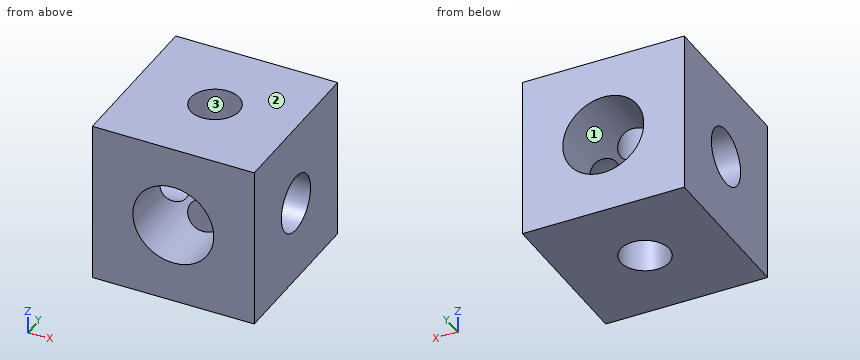
from build123d import *

# Parameters (mm, degrees)
F0_W     = 20
F0_H     = 20
F1_DEPTH = 20
F2_R     = 3
F3_DEPTH = 25
F4_R     = 3.5
F5_DEPTH = 25
F6_R     = 5
F7_DEPTH = 25


with BuildPart() as f1:
    # F0 (on Front) → F1 (new body)
    with BuildSketch(Plane.XZ):
        with Locations((15.513396, -6.90791)):
            Rectangle(F0_W, F0_H)
    extrude(amount=F1_DEPTH)

    # F2 (on face) → F3 (cut)
    with BuildSketch(Plane.XY.offset(3.09209)):
        with Locations((15.513396, -10)):
            Circle(F2_R)
    extrude(amount=-F3_DEPTH, mode=Mode.SUBTRACT)

    # F4 (on face) → F5 (cut)
    with BuildSketch(Plane.YZ.offset(25.513396)):
        with Locations((-10, -6.90791)):
            Circle(F4_R)
    extrude(amount=-F5_DEPTH, mode=Mode.SUBTRACT)

    # F6 (on face) → F7 (cut)
    with BuildSketch(Plane.XZ.offset(20)):
        with Locations((15.513396, -6.90791)):
            Circle(F6_R)
    extrude(amount=-F7_DEPTH, mode=Mode.SUBTRACT)


solid = f1.part
The model under review builds one solid part; all positions refer to its coordinate system, in mm. Face numbers are marked on the shaded views. Give positions to 0.01 mm unless a question says otherwise; leave off trailing zeros. Order: outer loops, then holes, each group sorted by start corner. A loop starts at its lowest first (then second) coordinate and runs counter-clockwise, first axis right, second up. Notation, with made-up numbers: M 80.5,70 L 111.5,70 A18 ccw 111.5,94 Z; hole C 44.5,-32.5 d11. An arc over 180 degrees is marked long. Use one line per item in the form item = value. Start each with the question number.
Item 1: To check wall thickness, follow line 1 along X through (y, z) = (-10, 1.75); line 2 along X through (y, z) = (-4.75, -6.75); line 3 along Z through (x, y) = (12.75, -13.75). State the ranges of each line that lie inside material, in increasing order. Write a range as from..to.
Item 2: Insertion check: pin 1 Ø7 at (x, y) = (15.51, -10) entering from -Z; pin 2 Ø8 at (x, z) = (15.51, -6.91) entering from -Y. Each pin has a flat end and moves straight along its axis. Give the tip position at first contact, or say it passes through.
Item 3: We need section A-A on y = -10. Give the boundary of the cut face in (x, z).
Item 4: We need section D-D on y = -7.5. Give the boundary of the cut face in (x, z).
Item 5: The part is to be moulded in two halves that separate along Z. For the marked faces 1, 2 and 3, say which applies: pulls with the +Z half, pulls with the -Z half, needs draft (parallel to the pull), parting line crosses it, or undercut.
Item 6: We need section C-C on z = -2.5. Give the boundary of the cut face in (x, y).
Item 7: We need section B-B on x = 17.75. Give the boundary of the cut face in (y, z), plus the area to 3 significant figures.
Completed:
q1.line_1 = 5.51..12.51, 18.51..25.51
q1.line_2 = 5.51..10.52, 20.51..25.51
q1.line_3 = -16.91..-11.07, -2.74..3.09
q2.pin_1 = -16.91
q2.pin_2 = through
q3.outline = M 5.51,-16.91 L 12.51,-16.91 L 12.51,-10.91 A5 cw 11.94,-10.41 L 5.51,-10.41 Z; M 5.51,-3.41 L 11.94,-3.41 A5 cw 12.51,-2.91 L 12.51,3.09 L 5.51,3.09 Z; M 18.51,-16.91 L 25.51,-16.91 L 25.51,-10.41 L 19.08,-10.41 A5 cw 18.51,-10.91 Z; M 18.51,-2.91 A5 cw 19.08,-3.41 L 25.51,-3.41 L 25.51,3.09 L 18.51,3.09 Z
q4.outline = M 5.51,-16.91 L 13.86,-16.91 L 13.86,-11.62 A5 cw 11.15,-9.36 L 5.51,-9.36 Z; M 5.51,-4.46 L 11.15,-4.46 A5 cw 13.86,-2.19 L 13.86,3.09 L 5.51,3.09 Z; M 17.17,-16.91 L 25.51,-16.91 L 25.51,-9.36 L 19.87,-9.36 A5 cw 17.17,-11.62 Z; M 17.17,-2.19 A5 cw 19.87,-4.46 L 25.51,-4.46 L 25.51,3.09 L 17.17,3.09 Z
q5.face_1 = undercut
q5.face_2 = pulls with the +Z half
q5.face_3 = needs draft
q6.outline = M 5.51,-20 L 13.15,-20 L 13.15,-11.85 A3 cw 13.15,-8.15 L 13.15,0 L 5.51,0 Z; M 17.87,-20 L 25.51,-20 L 25.51,0 L 17.87,0 L 17.87,-8.15 A3 cw 17.87,-11.85 Z
q7.outline = M -20,-16.91 L -12,-16.91 L -12,-11.38 L -20,-11.38 Z; M -20,-2.44 L -12,-2.44 L -12,3.09 L -20,3.09 Z; M -8,-16.91 L 0,-16.91 L 0,-11.38 L -8,-11.38 Z; M -8,-2.44 L 0,-2.44 L 0,3.09 L -8,3.09 Z
q7.area = 177 mm²
